For this review, take the finished solid that the model builds, in its own axes (mm). Round coordinates to 2 decimals unless told otherwise and drop trailing zeros. Order: outer loops, then holes, each group sorted by start corner. A loop starts at its lowest first (then second) coordinate and runs counter-clockwise, first axis right, second up.
from build123d import *

# Parameters (mm, degrees)
F0_R     = 20
F1_DEPTH = 4
F2_R     = 20
F2_R_2   = 18.25
F3_DEPTH = 80
F4_R     = 0.5
F5_R     = 3


with BuildPart() as f1:
    # F0 (on Top) → F1 (new body)
    with BuildSketch(Plane.XY):
        Circle(F0_R)
    extrude(amount=F1_DEPTH)

    # F2 (on face) → F3 (join)
    with BuildSketch(Plane.XY.offset(4)):
        Circle(F2_R)
        Circle(F2_R_2, mode=Mode.SUBTRACT)
    extrude(amount=F3_DEPTH)

    # F4
    f4_edges = [f1.edges().sort_by_distance(p)[0] for p in [
        (-18.25, 0, 84),
    ]]
    fillet(f4_edges, radius=F4_R)

    # F5
    f5_edges = [f1.edges().sort_by_distance(p)[0] for p in [
        (-20, 0, 0),
    ]]
    fillet(f5_edges, radius=F5_R)


solid = f1.part
(1) Add section C-C on z = 57. Give the boundary of the cut face in (x, y).
(2) Add section A-A on x = 0. Give the boundary of the cut face in (y, z), plus the area to 3 significant figures.
(3) Wall thickness on L1, parallel to Y at x = 0, z = 43.5; L2, parallel to Z at x = -6, y = 5; L3, parallel to Y at x = 5, z = 38: over which ranges is each line inside the solid? List them lowest first.
(4) Clearance check with flat-ended pins moving along their axes: P1, Ø1, axis at x = -1.5, z = 13.5, coming from the +Y side (3 decimals); P2, Ø5, axis at x = 9.5, y = -13, coming from the +Z side; P3, Ø6, axis at y = -7.5, z = 45, coming from the -X side. State where each tip first meets the part, or that it passes through.
(5) Draft analysis for pull direction Y (two halves, no side actions). For faces 1 (the face through (-3.956, -17.816, 43.194)), 2 (the face through (6, 18, 84)), 3 (the face through (-4.336, -19.524, 42.933)), 4 (the face through (0, 0, 4)), state which applies: pulls with the +Y half, pulls with the -Y half, needs draft (parallel to the pull), parting line crosses it, or undercut.
Here are the results:
1. outline: circle Ø40 at (0, 0); hole circle Ø36.5 at (0, 0)
2. outline: (-20, 3) arc R3 ccw to (-17, 0) - (17, 0) arc R3 ccw to (20, 3) - (20, 84) - (18.75, 84) arc R0.5 ccw to (18.25, 83.5) - (18.25, 4) - (-18.25, 4) - (-18.25, 83.5) arc R0.5 ccw to (-18.75, 84) - (-20, 84) - close
2. area: 436 mm2
3. L1: y = -20 to -18.25, 18.25 to 20
3. L2: z = 0 to 4
3. L3: y = -19.36 to -17.55, 17.55 to 19.36
4. P1: stops at y = 19.975
4. P2: stops at z = 83.98
4. P3: stops at x = -19.49
5. face 1: undercut
5. face 2: needs draft
5. face 3: parting line crosses it
5. face 4: undercut
